For this review, take the finished solid that the model builds, in its own axes (mm). Coordinates: 2 decimals unless noted, no trailing zeros. Loops run counter-clockwise (first coordinate to the right, second up) from the corner with the lowest first, then second, coordinate; pieces in that order, holes last. Notation, with made-up numbers: M -18.5,74 L 0.5,74 A30 cw 0.5,98 Z; hole C 25.25,2 d8. An arc over 180 degrees is marked long. Use one line per item in the form item = value.
```python
from build123d import *

# Parameters (mm, degrees)
BOSS_EXTRUDE1_DEPTH = 12.7


with BuildPart() as part:
    # Sketch1 → Boss-Extrude1 (new body, symmetric)
    with BuildSketch(Plane(origin=(0, 0, 0), x_dir=(0, 0, -1), z_dir=(1, 0, 0))):
        with BuildLine():
            Line((14.2875, 50.8), (50.8, 50.8))
            Line((50.8, 50.8), (50.8, 0))
            Line((50.8, 0), (-50.8, 0))
            Line((-50.8, 0), (-50.8, 50.8))
            Line((-50.8, 50.8), (-14.2875, 50.8))
            ThreePointArc((-14.2875, 50.8), (0, 36.5125), (14.2875, 50.8))
        make_face()
    extrude(amount=BOSS_EXTRUDE1_DEPTH, both=True)


solid = part.part
```
1. Wall thickness on line 1 along Z through (x, y) = (8.5, 48); line 2 along Z through (x, y) = (6, 41.5); line 3 along Y through (x, z) = (-8.5, -4.5): over which ranges is each line inside the solid? List them lowest first. Write a range as from..to.
Computed values:
line_1 = -50.8..-14.01, 14.01..50.8
line_2 = -50.8..-10.85, 10.85..50.8
line_3 = 0..37.24
2. For pin 1 Ø4 at (y, z) = (40.5, 0.5) entering from -X, flat-tipped, find the tip position at first contact; note if it passes through.
Computed values:
pin_1 = through
3. Consider section C-C on z = 0. Write out the cut boundary in (x, y).
Computed values:
outline = M -12.7,0 L 12.7,0 L 12.7,36.51 L -12.7,36.51 Z
4. Consider section B-B on x = -4.25. Write out the cut boundary in (y, z) (1 decimal), plus the area to 3 significant figures.
Computed values:
outline = M 0,-50.8 L 50.8,-50.8 L 50.8,-14.3 A14.3 cw 50.8,14.3 L 50.8,50.8 L 0,50.8 Z
area = 4,840 mm2
5. Consider section A-A on y = 44. Write out the cut boundary in (x, z).
Computed values:
outline = M -12.7,-50.8 L 12.7,-50.8 L 12.7,-12.57 L -12.7,-12.57 Z; M -12.7,12.57 L 12.7,12.57 L 12.7,50.8 L -12.7,50.8 Z
6. Draft analysis for pull direction Z (two halves, no side actions). For faces 1 (the face through (0.178, 36.516, 0.314)), 2 (the face through (0, 25, 50.8)), 3 (the face through (0, 50.8, 33)), state which applies: +Z half, -Z half, draft (parallel to the pull), parting line (faces both ways), or undercut.
Computed values:
face_1 = undercut
face_2 = +Z half
face_3 = draft
